```python
from build123d import *

# Parameters (mm, degrees)
CROQUIS1_R              = 4
SALIENTE_EXTRUIR1_DEPTH = 20
CHAFL_N1_SIZE           = 1
CORTAR_EXTRUIR2_DEPTH   = 0.25


with BuildPart() as part:
    # Croquis1 → Saliente-Extruir1 (new body)
    with BuildSketch(Plane(origin=(0, 0, 0), x_dir=(1, 0, 0), z_dir=(0, 1, 0))):
        Circle(CROQUIS1_R)
    extrude(amount=SALIENTE_EXTRUIR1_DEPTH)

    # Chaflán1
    chafl_n1_edges = [part.edges().sort_by_distance(p)[0] for p in [
        (-4, 0, 0),
        (-4, 20, 0),
    ]]
    chamfer(chafl_n1_edges, length=CHAFL_N1_SIZE)

    # Croquis4 → Cortar-Extruir2 (cut)
    with BuildSketch(Plane(origin=(0, 20, 0), x_dir=(1, 0, 0), z_dir=(0, 1, 0))):
        with BuildLine():
            add(Edge.make_bspline(
                [(-0.015518725, 2.134649306), (0.058547681, 2.13277333), (0.204020215, 2.129088757), (0.417820098, 2.100884068), (0.621928779, 2.052089336), (0.818008937, 1.98710307), (1.003715196, 1.900412344), (1.180445359, 1.795629318), (1.347778929, 1.671656222), (1.503460508, 1.529451391), (1.645925594, 1.374727444), (1.771440893, 1.209609832), (1.876632085, 1.035096915), (1.963015842, 0.851713109), (2.030785682, 0.659873146), (2.077550303, 0.458554285), (2.107422475, 0.249060925), (2.110914792, 0.10617308), (2.112686403, 0.033687768)],
                knots=[0, 0, 0, 0, 0.000222163, 0.000436347, 0.000645474, 0.000850973, 0.001054962, 0.001259031, 0.001466406, 0.001678557, 0.001890656, 0.002096587, 0.002299693, 0.002500778, 0.002703768, 0.002908812, 0.003119927, 0.003337287, 0.003337287, 0.003337287, 0.003337287], degree=3))
            add(Edge.make_bspline(
                [(2.112686403, 0.033687768), (2.110915051, -0.0382636), (2.107423512, -0.18008808), (2.077516338, -0.388252016), (2.030612338, -0.588355669), (1.963645177, -0.780064987), (1.877673201, -0.963582203), (1.771781577, -1.138424436), (1.647048765, -1.304649005), (1.505098078, -1.460434908), (1.35035403, -1.60328916), (1.184376582, -1.727767875), (1.010898502, -1.834881161), (0.827687407, -1.920348217), (0.63717308, -1.988658983), (0.437650425, -2.035233417), (0.230054363, -2.065275752), (0.088487501, -2.068725485), (0.016532557, -2.070478899)],
                knots=[0, 0, 0, 0, 0.000215759, 0.000425286, 0.000629551, 0.00083152, 0.00103333, 0.001236435, 0.001443647, 0.001655798, 0.001867897, 0.002074468, 0.002277305, 0.00247839, 0.002679869, 0.002883353, 0.003092087, 0.003307846, 0.003307846, 0.003307846, 0.003307846], degree=3))
            add(Edge.make_bspline(
                [(0.016532557, -2.070478899), (-0.055952379, -2.068708171), (-0.198839483, -2.065217595), (-0.408596095, -2.03529599), (-0.610056374, -1.988505928), (-0.802644204, -1.921638001), (-0.98646698, -1.835218309), (-1.161884218, -1.729841876), (-1.328191815, -1.604805143), (-1.484010953, -1.462900486), (-1.626581466, -1.308418712), (-1.750877895, -1.142893849), (-1.856278024, -0.969573328), (-1.942407547, -0.787976157), (-2.010595501, -0.598980223), (-2.057115293, -0.40132482), (-2.087213524, -0.196136813), (-2.09068192, -0.056430644), (-2.092441802, 0.014456999)],
                knots=[0, 0, 0, 0, 0.00021736, 0.000428475, 0.000634298, 0.000837024, 0.001038834, 0.001242626, 0.001449838, 0.001661989, 0.001874088, 0.002079537, 0.002281957, 0.002481593, 0.002681563, 0.002883489, 0.003089842, 0.003302399, 0.003302399, 0.003302399, 0.003302399], degree=3))
            add(Edge.make_bspline(
                [(-2.092441802, 0.014456999), (-2.09183079, 0.062037192), (-2.090616474, 0.156597333), (-2.075997397, 0.297016305), (-2.054784025, 0.435177056), (-2.024381839, 0.570686711), (-1.984619934, 0.703213551), (-1.937703331, 0.833671565), (-1.88040065, 0.960738678), (-1.815622767, 1.08501684), (-1.743323558, 1.204568733), (-1.663465558, 1.317573971), (-1.578853709, 1.424980824), (-1.486095545, 1.524005971), (-1.388248179, 1.61753015), (-1.283724318, 1.704116112), (-1.173161753, 1.784544628), (-1.056084748, 1.857025017), (-0.935378148, 1.922578314), (-0.810947544, 1.978831858), (-0.684482891, 2.027113071), (-0.555391865, 2.066245443), (-0.424017268, 2.097139198), (-0.290072372, 2.118176174), (-0.153663885, 2.132832537), (-0.061765234, 2.134041111), (-0.015518725, 2.134649306)],
                knots=[0, 0, 0, 0, 0.000142684, 0.000283569, 0.000423077, 0.000561875, 0.000699793, 0.000837942, 0.000977471, 0.001117606, 0.001258187, 0.001396235, 0.001532512, 0.001668024, 0.001802915, 0.001938339, 0.002074896, 0.002212747, 0.002351135, 0.002486682, 0.002622105, 0.002756954, 0.002891065, 0.003026617, 0.003163515, 0.003302194, 0.003302194, 0.003302194, 0.003302194], degree=3))
        make_face()
        with BuildLine():
            add(Edge.make_bspline(
                [(0.00210948, 1.724392896), (-0.035850101, 1.723930164), (-0.111406368, 1.723009125), (-0.223731552, 1.710876878), (-0.334579476, 1.693585577), (-0.443973033, 1.668920981), (-0.551454507, 1.63531635), (-0.658025754, 1.596641026), (-0.762714958, 1.549531208), (-0.86517651, 1.49630526), (-0.964508024, 1.437392208), (-1.058236826, 1.372281617), (-1.146605562, 1.302500412), (-1.229397867, 1.227885741), (-1.306370635, 1.148057625), (-1.379038865, 1.064226269), (-1.444489816, 0.973995536), (-1.504473332, 0.879812214), (-1.558150864, 0.781798979), (-1.605882698, 0.680987707), (-1.644927279, 0.576556065), (-1.676769995, 0.469637028), (-1.703169779, 0.360399931), (-1.719894263, 0.248016104), (-1.732159817, 0.133050262), (-1.733028212, 0.055356714), (-1.733467443, 0.016059563)],
                knots=[0, 0, 0, 0, 0.000113827, 0.000226566, 0.000338539, 0.000450309, 0.000562594, 0.000676167, 0.000790231, 0.000906707, 0.001022414, 0.001136438, 0.001248815, 0.001360011, 0.00147051, 0.001581322, 0.001692547, 0.001804581, 0.001916109, 0.00202759, 0.002138911, 0.002250197, 0.002362147, 0.002475703, 0.002590835, 0.002708667, 0.002708667, 0.002708667, 0.002708667], degree=3))
            add(Edge.make_bspline(
                [(-1.733467443, 0.016059563), (-1.732010458, -0.041725833), (-1.729144118, -0.155407581), (-1.704049752, -0.321999746), (-1.665396067, -0.482100645), (-1.608416219, -0.634834255), (-1.537158374, -0.781513436), (-1.449127642, -0.920836984), (-1.344831545, -1.052842554), (-1.226358943, -1.176608576), (-1.096847278, -1.28957521), (-0.959324158, -1.388733391), (-0.815262892, -1.472630819), (-0.664287804, -1.540979473), (-0.507204902, -1.595139174), (-0.343001986, -1.632257609), (-0.17277289, -1.656686701), (-0.056737855, -1.659032708), (0.00210948, -1.660222489)],
                knots=[0, 0, 0, 0, 0.000173262, 0.000340861, 0.0005043, 0.000666548, 0.000828884, 0.000992726, 0.001159918, 0.001332774, 0.001505994, 0.001674777, 0.001840658, 0.002005251, 0.002171224, 0.002338187, 0.002509641, 0.002686071, 0.002686071, 0.002686071, 0.002686071], degree=3))
            add(Edge.make_bspline(
                [(0.00210948, -1.660222489), (0.041663196, -1.659679055), (0.120110095, -1.658601263), (0.236790692, -1.647745632), (0.351369219, -1.630337782), (0.463684968, -1.605274175), (0.573610466, -1.573905939), (0.681604527, -1.536639965), (0.786516859, -1.49014716), (0.889670959, -1.438778073), (0.988409521, -1.380217893), (1.082667272, -1.31731715), (1.170068392, -1.247638727), (1.25279876, -1.174132655), (1.330087547, -1.095316829), (1.4014121, -1.011293718), (1.466532251, -0.921532967), (1.52649299, -0.827492504), (1.579982434, -0.729211072), (1.626587118, -0.628034297), (1.666125536, -0.524211315), (1.698043828, -0.417592376), (1.723055784, -0.308379978), (1.740289978, -0.196427888), (1.752345336, -0.081960068), (1.753253996, -0.004538519), (1.753712044, 0.03448905)],
                knots=[0, 0, 0, 0, 0.000118633, 0.000235285, 0.000351216, 0.000466113, 0.00058025, 0.000694035, 0.000808509, 0.000924255, 0.001039553, 0.001152673, 0.001263924, 0.001374585, 0.00148451, 0.001594802, 0.001704908, 0.001816941, 0.001929172, 0.002040317, 0.002150888, 0.002262174, 0.002373943, 0.002486708, 0.002601839, 0.00271887, 0.00271887, 0.00271887, 0.00271887], degree=3))
            add(Edge.make_bspline(
                [(1.753712044, 0.03448905), (1.753253629, 0.073249626), (1.752344279, 0.150138369), (1.740295736, 0.263807876), (1.723037576, 0.374954403), (1.69816591, 0.483141607), (1.666108591, 0.588397064), (1.626580213, 0.690621918), (1.579968443, 0.790196999), (1.526473329, 0.886876195), (1.466340959, 0.979647324), (1.400633253, 1.068335796), (1.328215712, 1.151276071), (1.251157398, 1.230515722), (1.167533529, 1.304364738), (1.077722907, 1.372847619), (0.982815847, 1.437617076), (0.882327578, 1.496046289), (0.778620202, 1.550005412), (0.67220425, 1.59623513), (0.564285279, 1.635517552), (0.455137722, 1.669022655), (0.34384289, 1.693488975), (0.2311528, 1.710892461), (0.117223361, 1.723004902), (0.040602539, 1.723928763), (0.00210948, 1.724392896)],
                knots=[0, 0, 0, 0, 0.00011623, 0.000230564, 0.000342537, 0.000453525, 0.000563278, 0.000672352, 0.000782043, 0.000892869, 0.001003554, 0.00111349, 0.001223695, 0.001333619, 0.001444879, 0.001558028, 0.00167226, 0.001789346, 0.001906533, 0.002022797, 0.002137122, 0.002250941, 0.002365055, 0.002478611, 0.002592945, 0.002708374, 0.002708374, 0.002708374, 0.002708374], degree=3))
        make_face(mode=Mode.SUBTRACT)
    extrude(amount=-CORTAR_EXTRUIR2_DEPTH, mode=Mode.SUBTRACT)


solid = part.part
```
Read the model definition and answer for the solid it produces. Units are mm, in the model's axes. Give positions to 0.01 mm unless a question says otherwise; leave off trailing zeros. Write each loop counter-clockwise with the first axis right and the second up, starting at its lowest first coordinate (ties: lowest second). Pieces come first, ordered by that corner, then holes. Notation, with made-up numbers: M 86.5,19 L 132.5,19 A23 ccw 132.5,58 Z; hole C 21.25,33 d2. An arc over 180 degrees is marked long. Put each result on its own line as item: value. Start each with the question number.
1. This flat-tipped pin is pushed along its axis until it touches: pin 1 Ø1.5 at (x, z) = (-2.5, -3) entering from -Y. Where does it stop, or does it pass through?
2. Consider line 1 along X through (y, z) = (1.75, 1); line 2 along X through (y, z) = (8.25, -2); line 3 along Y through (x, z) = (-3, 0.25). Determine where each line is inside the solid, lowest interval first.
3. The part is cut by section A-A, the plane y = 10.5. Give the vertices of the cut face in (x, z), and give its area (3 significant figures).
Final values:
1. pin 1: stops at y = 0.16
2. line 1: x = -3.87 to 3.87
2. line 2: x = -3.46 to 3.46
2. line 3: y = 0.01 to 19.99
3. outline: C 0,0 d8
3. area: 50.3 mm²
